Build history of the part. All positions in model axes, mm. A direction names the side the tool comes from. Coordinates: 2 decimals unless noted, no trailing zeros. Order: outer loops, then holes, each group sorted by start corner. A loop starts at its lowest first (then second) coordinate and runs counter-clockwise, first axis right, second up. Notation, with made-up numbers: (86.25, 19) - (104.25, 19) arc R17 ccw to (104.25, 31) - close; hole circle Ø9 at (83, 68.25). An arc over 180 degrees is marked (long way). One line per item, written item: value.
Autodesk Fusion 360 part; units mm, degrees
sketch "Schizzo1" plane through (0, 0, 0) normal (0, 0, 1) x (1, 0, 0)
  line L0 (0, 0) -> (31.5, 0)
  line L1 (31.5, 0) -> (31.5, 14)
  line L2 (31.5, 14) -> (0, 14)
  line L3 (0, 14) -> (0, 0)
  line L4 (0, 14) -> (0, 15.5)
  line L5 (0, 15.5) -> (31.5, 15.5)
  line L6 (0, 0) -> (0, -1.5)
  line L7 (0, -1.5) -> (31.5, -1.5)
  line L8 (33, 14) -> (33, 0)
  arc A0 (31.5, -1.5) -> (33, 0) centre (31.5, 0) ccw
  arc A1 (33, 14) -> (31.5, 15.5) centre (31.5, 14) ccw
  line L9 (0, 0) -> (-6.5, 0)
  line L10 (0, 14) -> (-6.5, 14)
  line L11 (-6.5, 14) -> (-6.5, 0)
  line L12 (0, -1.5) -> (-6.5, -1.5)
  line L13 (-6.5, -1.5) -> (-6.5, 0)
  line L14 (-6.5, 14) -> (-6.5, 15.5)
  line L15 (-6.5, 15.5) -> (0, 15.5)
  line L16 (-6.5, 15.5) -> (-16.5, 15.5)
  line L17 (-6.5, 0) -> (-16.5, 0)
  line L18 (-16.5, 15.5) -> (-16.5, 0)
  line L19 (-6.5, -1.5) -> (-16.5, -1.5)
  line L20 (-16.5, -1.5) -> (-16.5, 0)
  line L21 (-6.5, 14) -> (-16.5, 14)
  line L22 (-16.5, -1.5) -> (-16.5, -10.5)
  line L23 (0, -1.5) -> (0, -10.5)
  line L24 (0, -10.5) -> (-16.5, -10.5)
  line L25 (-16.5, 15.5) -> (-16.5, 24.5)
  line L26 (0, 15.5) -> (0, 24.5)
  line L27 (-16.5, 24.5) -> (0, 24.5)
  circle A2 centre (-8.25, -6) radius 1.5
  circle A3 centre (-8.25, 20) radius 1.5
  line L28 (31.5, 0) -> (24.5, 0)
  line L29 (24.5, 1) -> (31, 1)
  line L30 (24.5, 13) -> (31, 13)
  line L31 (31, 13) -> (31, 1)
  line L32 (24.5, 13) -> (24.5, 1)
  dimension "d1" = 31.5
  dimension "d2" = 14
  dimension "d3" = 1.5
  dimension "d4" = 1.5
  dimension "d5" = 1.5
  dimension "d6" = 1.5
  dimension "d7" = 1.5
  dimension "d8" = 1.5
  dimension "d9" = 6.5
  dimension "d10" = 6.5
  dimension "d11" = 10
  dimension "d12" = 10
  dimension "d13" = 9
  dimension "d14" = 9
  dimension "d15" = 9
  dimension "d16" = 9
  dimension "d17" = 3
  dimension "d18" = 3
  dimension "d19" = 7
  dimension "d20" = 1
  dimension "d21" = 6.5
  dimension "d23" = 6.5
extrude "Estrusione1" add sketch "Schizzo1" along normal blind 2 contours L0 L1 L2 L3 L28 makes body 1
extrude "Estrusione2" add sketch "Schizzo1" along normal blind 9 contours L0 L1 L2 L4 L5 L6 L7 L8 A0 A1 L28 bodies 1
extrude "Estrusione3" add sketch "Schizzo1" along normal blind 5 separate body contours L3 L9 L10 L11 makes body 2
extrude "Estrusione4" add sketch "Schizzo1" along normal blind 5 contours L6 L9 L12 L13 | L4 L10 L14 L15 | L12 L19 L22 L23 L24 | L11 L17 L18 L21 | L13 L17 L19 L20 | L15 L16 L25 L26 L27 | L14 L16 L18 L21 bodies 1 2
extrude "Estrusione5" add sketch "Schizzo1" along normal blind 5 contours A3 bodies 1
extrude "Estrusione6" add sketch "Schizzo1" along normal blind 5 contours A2 bodies 1
hole "Foratura1" at (-8.25, 20, 5) direction (0, 0, -1) diameter 2.529 depth 6 tip angle 118 bodies 1
hole "Foratura2" at (-8.25, -6.0001, 5) direction (0, 0, -1) diameter 2.529 depth 6 tip angle 118 bodies 1
1. Band-saw the part on C-C, the plane x = -8.25. Give the cut face in (y, z), and give its area (3 significant figures).
Values found:
outline: (-10.5, 0) - (-7.26, 0) - (-7.26, 5) - (-10.5, 5) - close; (-4.74, 0) - (18.74, 0) - (18.74, 5) - (-4.74, 5) - close; (21.26, 0) - (24.5, 0) - (24.5, 5) - (21.26, 5) - close
area: 150 mm2
2. 3-axis set-ups, long thin cutter, end or side, ignore diameter. For faces 4 (the face through (28, 1, 1)), 5 (the face through (31.5, 7, 5)), 6 (the face through (16, 15.5, 4)), 7 (the face through (0, -1, 7)): which of +Z, -Z, +X, -X, +Y, -Y reach the whole face in a straight line?
Values found:
face 4: +Z, -Z
face 5: +Z
face 6: +Z, -Z, +X, +Y
face 7: +Z, -X, +Y, -Y
3. Two-plate mould, pull along X, no slides. Class faces 1 (the face through (32.55, 15.07, 4.44)), 2 (the face through (-8, 7, 5)), 3 (the face through (-7.016, -5.726, 2.465)): pulls with the +X half, pulls with the -X half, needs draft (parallel to the pull), parting line crosses it, or undercut.
Values found:
face 1: pulls with the +X half
face 2: needs draft
face 3: undercut
4. Band-saw the part on B-B, the plane y = 9.5. Give the cut face in (x, z).
Values found:
outline: (-16.5, 0) - (24.5, 0) - (24.5, 2) - (0, 2) - (0, 5) - (-16.5, 5) - close; (31, 0) - (33, 0) - (33, 9) - (31.5, 9) - (31.5, 2) - (31, 2) - close
5. Probe line 1 along Y through (x, z) = (-8.25, 2.9); line 2 along X through (y, z) = (20, 2.45); line 3 along Y through (x, z) = (10, 4). List the from-to ranges inside material, lowest first.
Values found:
line 1: y = -10.5 to -7.26, -4.74 to 18.74, 21.26 to 24.5
line 2: x = -16.5 to -9.51, -6.99 to 0
line 3: y = -1.5 to 0, 14 to 15.5
6. Band-saw the part on D-D, the plane z = 6.5. Give the cut face in (x, y), and give its area (3 significant figures).
Values found:
outline: (0, -1.5) - (31.5, -1.5) arc R1.5 ccw to (33, 0) - (33, 14) arc R1.5 ccw to (31.5, 15.5) - (0, 15.5) - (0, 14) - (31.5, 14) - (31.5, 0) - (0, 0) - close
area: 119 mm2
7. Flat gauge pins, fed straight in: P1, Ø3, axis at x = 14, z = 2, coming from the -Y side; P2, Ø1.2, axis at y = 15, z = 7, coming from the -X side; P3, Ø2, axis at x = 9.5, z = 6, coming from the +Y side; P4, Ø1.5, axis at x = -8.25, y = -6, coming from the -Z side. Where does each tip first touch, or does it go through?
Values found:
P1: stops at y = -1.5
P2: stops at x = 0
P3: stops at y = 15.5
P4: passes through
8. Band-saw the part on A-A, the plane x = 29. Give the cut face in (y, z).
Values found:
outline: (-1.5, 0) - (1, 0) - (1, 2) - (0, 2) - (0, 9) - (-1.5, 9) - close; (13, 0) - (15.5, 0) - (15.5, 9) - (14, 9) - (14, 2) - (13, 2) - close
